Part model, mm, in its own coordinate system. Face numbers are marked on the shaded views. A direction names the side the tool comes from. Round coordinates to 2 decimals unless told otherwise and drop trailing zeros. Write each loop counter-clockwise with the first axis right and the second up, starting at its lowest first coordinate (ties: lowest second). Pieces come first, ordered by that corner, then holes. Notation, with made-up numbers: (16.25, -26.5) -> (64.25, -26.5) arc R22 ccw to (64.25, 0.5) -> close; hole circle Ø4 at (2, 33.25). An arc over 180 degrees is marked (long way). Return JSON: item names as keys, results as strings. Group by question number.
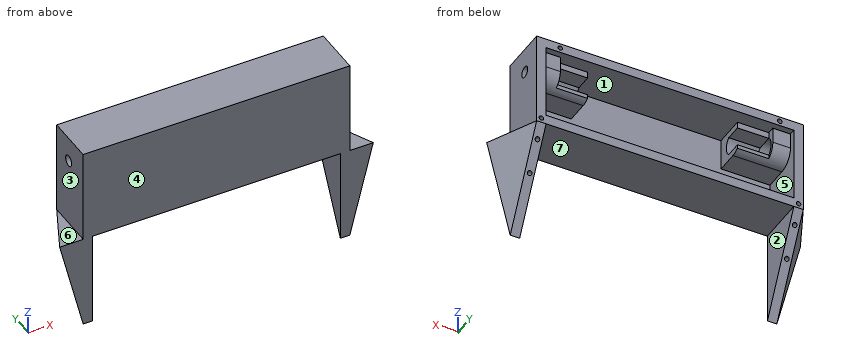
Autodesk Inventor part; units mm, degrees
ref_plane "Work Plane2" through (85, 31, -30) normal (-0.8782, -0.4249, 0.2195) x (0, -0.459, -0.8884)
ref_plane "YZ Plane" through (0, 0, 0) normal (1, 0, 0) x (0, 1, 0)
ref_plane "XZ Plane" through (0, 0, 0) normal (0, 1, 0) x (-1, 0, 0)
sketch "Sketch1" plane through (0, 0, 0) normal (0, 1, 0) x (-1, 0, 0)
  line L0 (85, 30) -> (-85, 30)
  line L1 (-85, 30) -> (-85, -30)
  line L2 (-85, -30) -> (85, -30)
  line L3 (85, -30) -> (85, 30)
  line L4 (85, 30) -> (-85, -30) construction
  line L5 (-85, 30) -> (85, -30) construction
  line L6 (0, -42) -> (0, 42)
  point P0 (0, 0)
  point P1 (-100, -30)
  point P2 (-85, -27)
  dimension "d0" = 170
  dimension "d1" = 60
  dimension "d32" = 15
extrude "Extrusion1" add sketch "Sketch1" along normal blind 3
sketch "Sketch2" plane through (0, 3, 0) normal (0, 1, 0) x (1, 0, 0)
  line L0 (-85, 30) -> (-85, -30)
  line L1 (-85, -30) -> (85, -30)
  line L2 (85, -30) -> (85, 30)
  line L3 (79, -24) -> (-79, -24)
  line L4 (-79, -24) -> (-79, 24)
  line L5 (-79, 24) -> (79, 24)
  line L6 (79, 24) -> (79, -24)
  line L7 (79, -24) -> (-79, 24) construction
  line L8 (-79, -24) -> (79, 24) construction
  line L9 (85, 30) -> (-85, 30)
  point P0 (0, 0)
  dimension "d36" = 158
  dimension "d37" = 48
extrude "Extrusion2" add sketch "Sketch2" along normal blind 28
sketch "Sketch7" plane through (-79, 3, 24) normal (1, 0, 0) x (0, 0, -1)
  circle A0 centre (10, 14) radius 8
  line L0 (54, -3) -> (-6, -3)
  circle A1 centre (10, 14) radius 10
  line L1 (0, 14) -> (0, 0)
  line L2 (0, 14) -> (20, 14)
  line L3 (20, 14) -> (20, 0)
  line L4 (-6, -3) -> (-6, 28)
  line L5 (0, 0) -> (20, 0)
  line L6 (10, 24) -> (0, 24)
  line L7 (0, 0) -> (0, 28)
  line L8 (0, 14) -> (0, 24)
  point P0 (24, -3)
  point P1 (54, -3)
  dimension "MotorDiameter" = 16
  dimension "d18" = 17
  dimension "d20" = 2
  dimension "d40" = 20
  dimension "d62" = 10
extrude "Extrusion5" add sketch "Sketch7" along normal blind 11.25 contours L2 A1 A0 | A0 L2 A1 | L3 L5 L1 A1 | L7 L6 A1
sketch "Sketch8" plane through (-67.75, 3, 24) normal (1, 0, 0) x (0, 0, -1)
  arc A0 (20, 14) -> (10, 24) centre (10, 14) ccw
  circle A1 centre (10, 14) radius 8
  line L0 (0, 0) -> (0, 24)
  line L1 (20, 0) -> (0, 0)
  line L2 (20, 0) -> (20, 14)
  circle A2 centre (10, 14) radius 7.75
  line L3 (10, 24) -> (0, 24)
  line L4 (0, 0) -> (0, 24)
  line L5 (4, 9.0946) -> (4, 19.2915)
  line L6 (10, 24) -> (0, 24)
  line L7 (16, 9.0946) -> (16, 19.2915)
  line L8 (16, 19.2915) -> (18.4853, 19.2915)
  arc A3 (20, 14) -> (10, 24) centre (10, 14) ccw
  line L9 (4, 19.2915) -> (0, 19.2915)
  point P0 (24, -3)
  point P1 (4, 27)
  point P2 (4, 18.9054)
  point P3 (16, 18.9054)
  dimension "d55" = 15.5
  dimension "d63" = 12
  dimension "d64" = 6
extrude "Extrusion6" add sketch "Sketch8" along normal blind 20 contours L2 L1 L0 L9 A1 L8 A0 | A1 L5 A2 L7 | A2 L7 | L5 A2 picked at (9.114, 6.2488)
sketch "Sketch9" plane through (-79, 20, 20) normal (1, 0, 0) x (0, 0, -1)
  circle A0 centre (6, -3) radius 3.5
  line L0 (50, -20) -> (-10, -20)
  line L1 (-10, -20) -> (-10, 11)
  point P0 (20, -20)
  point P1 (44, -20)
  dimension "d27" = 7
  dimension "d28" = 17
  dimension "d41" = 16
extrude "Extrusion7" cut sketch "Sketch9" against normal up to surface (6 mm away)
mirror "Mirror2" about plane through (0, 0, 0) normal (1, 0, 0) of "Extrusion7", "Extrusion6", "Extrusion5"
sketch "Sketch15" plane through (85, 0, 30) normal (1, 0, 0) x (0, 0, -1)
  line L0 (60, 31) -> (0, 31)
  line L1 (60, 31) -> (120, 0)
  line L2 (120, 0) -> (60, 0)
  circle A0 centre (16, 17) radius 3.5
  line L3 (0, 0) -> (60, 0)
  line L4 (60, 0) -> (60, 31)
  line L5 (0, 31) -> (60, 31)
  line L6 (0, 0) -> (0, 31)
  point P0 (30, 0)
  dimension "d67" = 60
extrude "Extrusion12" add sketch "Sketch15" against normal blind 6 contours L1 L2 L4
mirror "Mirror5" about plane through (0, 0, 0) normal (1, 0, 0) of "Extrusion12"
sketch "Sketch16" plane through (79, 0, -30) normal (0, 0, -1) x (-1, 0, 0)
  line L0 (-6, 0) -> (-6, 31)
  line L1 (-6, 0) -> (0, 0)
  line L2 (0, 31) -> (0, 0)
  line L3 (-6, 31) -> (0, 31)
  line L4 (200.8, 0) -> (-56.8, 0)
  line L5 (-6, 31) -> (-21, 0)
  line L6 (-6, 0) -> (-21, 0)
  point P0 (79, 0)
  dimension "SideOffset" = 15
extrude "Extrusion13" add sketch "Sketch16" along normal blind 60 contours L4 L5 L0
ref_plane "Work Plane2" through (85, 31, -30) normal (-0.8782, -0.4249, 0.2195) x (0, -0.459, -0.8884)
sketch "Sketch19" plane through (85, 31, -30) normal (-0.8782, -0.4249, 0.2195) x (0, -0.459, -0.8884)
  line L0 (-86.7961, -100.9494) -> (167.9591, -100.9494)
  line L1 (167.9591, -100.9494) -> (167.9591, 132.7149)
  line L2 (167.9591, 132.7149) -> (-86.7961, 132.7149)
  line L3 (-86.7961, 132.7149) -> (-86.7961, -100.9494)
  point P0 (-12.4232, -4.3756)
extrude "Extrusion14" cut sketch "Sketch19" against normal blind 60
mirror "Mirror8" about plane through (0, 0, 0) normal (1, 0, 0) of "Extrusion13", "Extrusion14"
sketch "Sketch20" plane through (79, 0, -90) normal (0, 0.8884, -0.459) x (1, 0, 0)
  line L0 (6, 0) -> (6, -67.5352)
  line L1 (6, 0) -> (0, 0)
  line L2 (0, -67.5352) -> (0, 0)
  line L3 (6, -67.5352) -> (0, -67.5352)
  line L4 (-164, 0) -> (-164, -67.5352)
  line L5 (-158, -67.5352) -> (-164, -67.5352)
  line L6 (-158, -67.5352) -> (-158, 0)
  line L7 (-164, 0) -> (-158, 0)
  circle A0 centre (3, -57.5352) radius 1.45
  line L8 (6, -67.5352) -> (0, -67.5352)
  line L9 (3, -67.5352) -> (3, 0)
  circle A1 centre (3, -37.5352) radius 1.45
  line L10 (-79, 24.6917) -> (-79, -148.1499)
  circle A2 centre (-161, -57.5352) radius 1.45
  circle A3 centre (-161, -37.5352) radius 1.45
  point P0 (-79, -79.9583)
  dimension "d75" = 2.9
  dimension "d76" = 10
  dimension "d77" = 2.9
  dimension "d78" = 20
extrude "Extrusion15" cut sketch "Sketch20" against normal blind 6.5 contours A1 L9 | L9 A1 | L9 A0 | A0 L9 | A2 | A3
sketch "Sketch21" plane through (0, 31, 0) normal (0, 1, 0) x (1, 0, 0)
  line L0 (85, -30) -> (85, 30)
  line L1 (85, 30) -> (79, 30)
  line L2 (79, 30) -> (-79, 30)
  line L3 (-79, 30) -> (-85, 30)
  line L4 (-85, 30) -> (-85, -30)
  line L5 (-85, -30) -> (85, -30)
  line L6 (79, 24) -> (79, -24)
  line L7 (79, -24) -> (-79, -24)
  line L8 (-79, -24) -> (-79, 24)
  line L9 (-79, 24) -> (79, 24)
  line L10 (82, -30) -> (82, 30)
  line L11 (85, 30) -> (79, 30)
  line L12 (85, -30) -> (85, 30)
  line L13 (85, -27) -> (-85, -27)
  line L14 (-85, 30) -> (-85, -30)
  line L15 (85, 27) -> (-85, 27)
  circle A0 centre (82, 27) radius 1.45
  line L16 (0, 42) -> (0, -42)
  circle A1 centre (-82, 27) radius 1.45
  circle A2 centre (70, -27) radius 1.45
  circle A3 centre (-70, -27) radius 1.45
  point P0 (0, 0)
  dimension "d82" = 3
  dimension "d83" = 3
  dimension "d84" = 3
  dimension "d85" = 2.9
  dimension "d86" = 2.9
  dimension "d87" = 15
extrude "Extrusion16" cut sketch "Sketch21" against normal blind 6.5 contours A0 L10 L15 | L15 L10 A0 | A0 L15 L10 | A2 L13 | L13 A2 | L15 A0 L10 | A3 L13 | L13 A3 | A1 L15 | L15 A1
ref_plane "Work Plane3" through (-85, 31, -30) normal (-0.8782, 0.4249, -0.2195) x (0, -0.459, -0.8884)
equation "\"d0\" = Width"
equation "\"d1\" = Length"
equation "\"d2\" = BaseWallThickness"
equation "\"d36\" = Width - 2 * SideWallThickness"
equation "\"d37\" = Length - 2 * SideWallThickness"
equation "\"d5\" = Height - 2 * BaseWallThickness"
equation "\"d18\" = DriveMotorHeight"
equation "\"d20\" = DriveMotorMountThickness"
equation "\"d28\" = DriveMotorHeight"
equation "\"d41\" = SideWallThickness + DriveMotorMountThickness + 0.5 * MotorDiameter"
equation "\"d67\" = WedgeLength"
equation "\"d68\" = SideWallThickness"
equation "\"SideOffset\" = SideTriangleWidth"
equation "\"d71\" = WedgeLength"
equation "\"d73\" = WedgeLength"
equation "\"d75\" = ScrewHoleDia"
equation "\"d77\" = ScrewHoleDia"
equation "\"d79\" = ScrewDepth"
equation "\"d82\" = 0.5 * SideWallThickness"
equation "\"d83\" = 0.5 * SideWallThickness"
equation "\"d84\" = 0.5 * SideWallThickness"
equation "\"d85\" = ScrewHoleDia"
equation "\"d86\" = ScrewHoleDia"
equation "\"d88\" = ScrewDepth"
equation "\"SideWallThickness\" = 6"
equation "\"BaseWallThickness\" = 3"
equation "\"Width\" = 170"
equation "\"Length\" = 60"
equation "\"Height\" = 34"
equation "\"DriveMotorHeight\" = 17"
equation "\"DriveMotorMountThickness\" = 2"
equation "\"WedgeLength\" = 60"
equation "\"SideTriangleWidth\" = 15"
equation "\"ScrewHoleDia\" = 2.9"
equation "\"ScrewDepth\" = 6.5"
properties part number "BodyWedgeV2" material "Thermoplastic Resin"
Item 1: Cut at A-A (z = -76). Write the cut outline in (x, y), then the cut area to 3 significant figures.
Item 2: Wall check: L1, parallel to X at y = 26.5, z = -27; L2, parallel to Z at x = -69, y = 17; L3, parallel to Z at x = 4, y = 23. Give the ranges that are in metal, low to high.
Item 3: Which spindle directions (+Z, -Z, +X, -X, +Y, -Y) get a long thin tool onto all of the face, cutting with end or side? Do the marked faces 1, 2 and 3. Say none if no direction does.
Item 4: Cut at D-D (x = 53). Write the cut outline in (y, z).
Item 5: Flat gauge pins, fed straight in: P1, Ø4, axis at y = 18, z = 16.5, coming from the +X side; P2, Ø1, axis at x = 21.5, y = 18, coming from the -Z side; P3, Ø10, axis at x = -51, z = 15.5, coming from the +Y side. Where does each tip first touch, or does it go through?
Item 6: Cut at C-C (y = 6.5). Write the cut outline in (x, z), then the cut area to 3 significant figures.
Item 7: Cut at B-B (x = -43). Write the cut outline in (y, z), then the cut area to 3 significant figures.
Item 8: Two-plate mould, pull along Z, no slides. Class the marked faces 4, 5, 6 and 7: released by +Z, released by -Z, zero draft, split by the parting line, or undercut.
Checks:
{
 "1": {"outline": "(-88.5, 0) -> (-79, 0) -> (-79, 7.23) -> (-85, 7.23) -> close; (79, 0) -> (88.5, 0) -> (85, 7.23) -> (79, 7.23) -> close", "area": "112 mm2"},
 "2": {"L1": "x = -85 to -83.45, -80.55 to 80.55, 83.45 to 85", "L2": "z = -30 to -24, 4 to 6, 22 to 30", "L3": "z = -30 to -24, 24 to 30"},
 "3": {"face 1": "+Y", "face 2": "-Z, +Y, -Y", "face 3": "+Z, -X, +Y, -Y"},
 "4": {"outline": "(0, -30) -> (31, -30) -> (31, -24) -> (3, -24) -> (3, 4) -> (17, 4) arc R10 ccw to (22.29, 5.51) -> (22.29, 8) -> (12.09, 8) arc R7.75 cw to (12.09, 20) -> (22.29, 20) -> (22.29, 24) -> (31, 24) -> (31, 30) -> (0, 30) -> close"},
 "5": {"P1": "stops at x = 85", "P2": "stops at z = -30", "P3": "stops at y = 22.29"},
 "6": {"outline": "(-96.85, -30) -> (-85, -77.42) -> (-79, -77.42) -> (-79, -30) -> (79, -30) -> (79, -77.42) -> (85, -77.42) -> (96.85, -30) -> (85, -30) -> (85, 30) -> (-85, 30) -> (-85, -30) -> close; hole (-79, -24) -> (79, -24) -> (79, 4) -> (47.75, 4) -> (47.75, 24) -> (-47.75, 24) -> (-47.75, 4) -> (-79, 4) -> close", "area": "5,000 mm2"},
 "7": {"outline": "(0, -30) -> (31, -30) -> (31, -24) -> (3, -24) -> (3, 24) -> (31, 24) -> (31, 30) -> (0, 30) -> close", "area": "516 mm2"},
 "8": {"face 4": "zero draft", "face 5": "undercut", "face 6": "released by +Z", "face 7": "released by -Z"}
}
